Check sheet for the modelled part. Datum: model origin and axes. Units: mm. Face numbers are marked on the shaded views. Coordinates: 2 decimals unless noted, no trailing zeros.
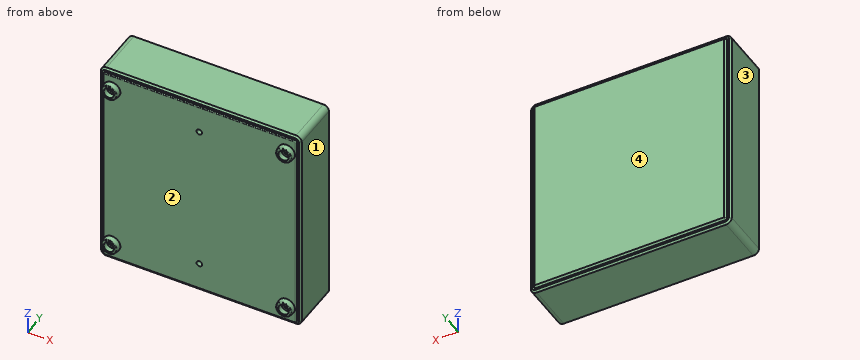
from build123d import *

# Parameters (mm, degrees)
SKETCH1_W                    = 107.6
SKETCH1_H                    = 114.4
BOSS_EXTRUDE1_DEPTH          = 30
SKETCH2_R                    = 1.5
CUT_EXTRUDE1_DEPTH           = 10
SKETCH3_R                    = 4.5
SKETCH3_R_2                  = 2.75
BOSS_EXTRUDE2_DEPTH          = 3
FILLET5_R                    = 0.5
FILLET5_OF_SKETCH_PATTERN1_R = 0.5
FILLET2_R                    = 3
SKETCH6_OUTSIDE_W            = 141.696
SKETCH6_OUTSIDE_H            = 148.496
CUT_EXTRUDE2_DEPTH           = 1
SKETCH7_OUTSIDE_W            = 141.696
SKETCH7_OUTSIDE_H            = 148.496
CUT_EXTRUDE3_DEPTH           = 1
CHAMFER1_SIZE                = 1
CHAMFER2_SIZE                = 1
FILLET4_R                    = 0.5


with BuildPart() as part:
    # Sketch1 → Boss-Extrude1 (new body)
    with BuildSketch(Plane(origin=(0, 0, 0), x_dir=(1, 0, 0), z_dir=(0, 1, 0))):
        with Locations((53.8, 57.2)):
            Rectangle(SKETCH1_W, SKETCH1_H)
    extrude(amount=BOSS_EXTRUDE1_DEPTH)

    # Sketch2 → Cut-Extrude1 (cut)
    with BuildSketch(Plane.XZ):
        with Locations(Location((7, -104, 0), (0, 0, 270))):
            Circle(SKETCH2_R)
        with Locations(Location((100.6, -104, 0), (0, 0, 270))):
            Circle(SKETCH2_R)
        with Locations(Location((100.6, -10.4, 0), (0, 0, 270))):
            Circle(SKETCH2_R)
        with Locations(Location((7, -10.4, 0), (0, 0, 270))):
            Circle(SKETCH2_R)
        with Locations(Location((53.8, -17.2, 0), (0, 0, 270))):
            Circle(SKETCH2_R)
        with Locations(Location((53.8, -97.2, 0), (0, 0, 270))):
            Circle(SKETCH2_R)
    extrude(amount=-CUT_EXTRUDE1_DEPTH, mode=Mode.SUBTRACT)

    # Sketch3 → Boss-Extrude2 (add)
    with BuildSketch(Plane.XZ):
        with Locations(Location((7, -104, 0), (0, 0, 270))):
            Circle(SKETCH3_R)
        with Locations(Location((7, -104, 0), (0, 0, 270))):
            Circle(SKETCH3_R_2, mode=Mode.SUBTRACT)
    boss_extrude2 = extrude(amount=BOSS_EXTRUDE2_DEPTH)

    # Sketch8 → Cut-Revolve1 (revolve, cut)
    with BuildSketch(Plane(origin=(7, 0, 0), x_dir=(0, 0, -1), z_dir=(1, 0, 0))):
        with BuildLine():
            Line((108.5, 0), (108.5, -3))
            Line((108.5, -3), (108, -3))
            ThreePointArc((108, -3), (108.374143795, -1.520690633), (108.5, 0))
        make_face()
    cut_revolve1 = revolve(axis=Axis((7, -3, -104), (0, 1, 0)), mode=Mode.SUBTRACT)

    # Fillet5
    fillet5_edges = [part.edges().sort_by_distance(p)[0] for p in [
        (7, -3, -100),
    ]]
    fillet(fillet5_edges, radius=FILLET5_R)

    # Sketch-Pattern1: Boss-Extrude2, Cut-Revolve1 at 3 more places
    with Locations((0, 0, 93.6), (93.6, 0, 93.6), (93.6, 0, 0)):
        add(boss_extrude2)
        add(cut_revolve1, mode=Mode.SUBTRACT)

    # Fillet5 of Sketch-Pattern1
    fillet5_of_sketch_pattern1_edges = [part.edges().sort_by_distance(p)[0] for p in [
        (7, -3, -6.4),
        (100.6, -3, -6.4),
        (100.6, -3, -100),
    ]]
    fillet(fillet5_of_sketch_pattern1_edges, radius=FILLET5_OF_SKETCH_PATTERN1_R)

    # Fillet2
    fillet2_edges = [part.edges().sort_by_distance(p)[0] for p in [
        (0, 15, -114.4),
        (107.6, 15, -114.4),
        (107.6, 15, 0),
        (0, 15, 0),
    ]]
    fillet(fillet2_edges, radius=FILLET2_R)

    # Sketch6 outside → Cut-Extrude2 (cut)
    with BuildSketch(Plane(origin=(0, 30, 0), x_dir=(1, 0, 0), z_dir=(0, 1, 0))):
        with Locations((53.8, 57.2)):
            Rectangle(SKETCH6_OUTSIDE_W, SKETCH6_OUTSIDE_H)
        with BuildLine():
            Line((2, 111.4), (2, 3))
            ThreePointArc((2, 3), (2.292893219, 2.292893219), (3, 2))
            Line((3, 2), (104.6, 2))
            ThreePointArc((104.6, 2), (105.307106781, 2.292893219), (105.6, 3))
            Line((105.6, 3), (105.6, 111.4))
            ThreePointArc((105.6, 111.4), (105.307106781, 112.107106781), (104.6, 112.4))
            Line((104.6, 112.4), (3, 112.4))
            ThreePointArc((3, 112.4), (2.292893219, 112.107106781), (2, 111.4))
        make_face(mode=Mode.SUBTRACT)
    extrude(amount=-CUT_EXTRUDE2_DEPTH, mode=Mode.SUBTRACT)

    # Sketch7 outside → Cut-Extrude3 (cut)
    with BuildSketch(Plane.XZ):
        with Locations((53.8, -57.2)):
            Rectangle(SKETCH7_OUTSIDE_W, SKETCH7_OUTSIDE_H)
        with BuildLine():
            Line((105.6, -111.4), (105.6, -3))
            ThreePointArc((105.6, -3), (105.307106781, -2.292893219), (104.6, -2))
            Line((104.6, -2), (3, -2))
            ThreePointArc((3, -2), (2.292893219, -2.292893219), (2, -3))
            Line((2, -3), (2, -111.4))
            ThreePointArc((2, -111.4), (2.292893219, -112.107106781), (3, -112.4))
            Line((3, -112.4), (104.6, -112.4))
            ThreePointArc((104.6, -112.4), (105.307106781, -112.107106781), (105.6, -111.4))
        make_face(mode=Mode.SUBTRACT)
    extrude(amount=-CUT_EXTRUDE3_DEPTH, mode=Mode.SUBTRACT)

    # Chamfer1
    chamfer1_edges = [part.edges().sort_by_distance(p)[0] for p in [
        (0.878679656, 29, -0.878679656),
        (53.8, 29, -114.4),
        (0, 29, -57.2),
        (53.8, 29, 0),
        (107.6, 29, -57.2),
        (106.721320344, 29, -113.521320344),
        (106.721320344, 29, -0.878679656),
        (0.878679656, 29, -113.521320344),
        (0.878679656, 1, -0.878679656),
        (107.6, 1, -57.2),
        (53.8, 1, 0),
        (0, 1, -57.2),
        (53.8, 1, -114.4),
        (106.721320344, 1, -113.521320344),
        (0.878679656, 1, -113.521320344),
        (106.721320344, 1, -0.878679656),
    ]]
    chamfer(chamfer1_edges, length=CHAMFER1_SIZE)

    # Chamfer2
    chamfer2_edges = [part.edges().sort_by_distance(p)[0] for p in [
        (53.8, 30, -112.4),
        (2.292893219, 30, -112.107106781),
        (105.307106781, 30, -112.107106781),
        (2, 30, -57.2),
        (105.6, 30, -57.2),
        (2.292893219, 30, -2.292893219),
        (105.307106781, 30, -2.292893219),
        (53.8, 30, -2),
    ]]
    chamfer(chamfer2_edges, length=CHAMFER2_SIZE - 0.0001)  # a hair under: the kernel refuses the full size

    # Fillet4
    fillet4_edges = [part.edges().sort_by_distance(p)[0] for p in [
        (105.307106781, 0, -2.292893219),
        (105.6, 0, -57.2),
        (105.307106781, 0, -112.107106781),
        (53.8, 0, -112.4),
        (2.292893219, 0, -112.107106781),
        (2, 0, -57.2),
        (2.292893219, 0, -2.292893219),
        (53.8, 0, -2),
    ]]
    fillet(fillet4_edges, radius=FILLET4_R - 0.0001)  # a hair under: the kernel refuses the full size


solid = part.part
(1) Release check for a two-part mould opening along X. For the marked faces 1, 2, 3 and 4 record: +X half, -X half, draft (parallel to the pull), parting line (faces both ways), or undercut.
Filled in:
face 1: +X half
face 2: undercut
face 3: -X half
face 4: draft
(2) Go/stop test with flat-tipped pins: P1, Ø6, axis at x = 100, z = -104, coming from the -Y side; P2, Ø0.6, axis at x = 31, y = 1, coming from the -Z side; P3, Ø3.5, axis at x = 100.6, z = -104, coming from the -Y side; P4, Ø0.6, axis at y = 0.5, z = -59.5, coming from the -X side. Record where each tip stops, or that it passes through.
Filled in:
P1: stops at y = -3
P2: stops at z = -113.7
P3: stops at y = 0
P4: stops at x = 2
(3) Thickness scan on probe 1 along X at (y, z) = (-1.25, -10.4); probe 2 along X at (y, z) = (4, -10); probe 3 along X at (y, z) = (-2.3, -104). Record the ranges inside material, lowest first.
Filled in:
probe 1: x = 2.58 to 4.25, 9.75 to 11.42, 96.18 to 97.85, 103.35 to 105.02
probe 2: x = 0 to 5.55, 8.45 to 99.15, 102.05 to 107.6
probe 3: x = 2.79 to 4.25, 9.75 to 11.21, 96.39 to 97.85, 103.35 to 104.81
